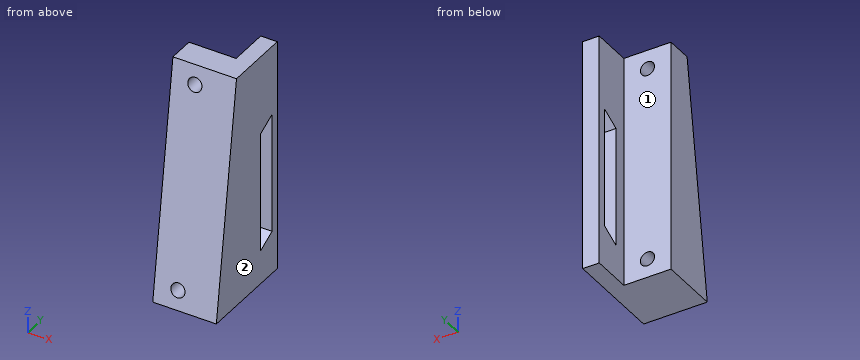
Autodesk Inventor part; units mm, degrees
ref_plane "YZ Plane" through (0, 0, 0) normal (1, 0, 0) x (0, 1, 0)
ref_plane "XZ Plane" through (0, 0, 0) normal (0, 1, 0) x (-1, 0, 0)
ref_plane "XY Plane" through (0, 0, 0) normal (0, 0, 1) x (1, 0, 0)
sketch "Sketch1" plane through (0, 0, 0) normal (0, 1, 0) x (-1, 0, 0)
  line L0 (0, 0) -> (20, 0)
  line L1 (20, 0) -> (20, -99)
  line L2 (20, -99) -> (0, -99)
  line L3 (0, -99) -> (0, 0)
  line L4 (10, 0) -> (10, -8)
  circle A0 centre (10, -8) radius 3
  line L5 (10, -99) -> (10, -91)
  circle A1 centre (10, -91) radius 3
  line L6 (0, -99) -> (-7, -99)
  line L7 (-7, -99) -> (-7, 0)
  line L8 (-7, 0) -> (0, 0)
  line L9 (0, 0) -> (0, -99)
  dimension "d0" = 20
  dimension "d1" = 99
  dimension "d2" = 8
  dimension "d3" = 6
  dimension "d4" = 8
  dimension "d5" = 6
  dimension "d8" = 7
extrude "Extrusion1" add sketch "Sketch1" along normal blind 25 contours L0 L1 L2 L3
extrude "Extrusion2" add sketch "Sketch1" along normal blind 42 contours L3 L6 L7 L8
sketch "Sketch2" plane through (0, 25, 0) normal (-1, 0, 0) x (0, 0, 1)
  line L0 (-84.6677, 5.4134) -> (-33.6677, 5.4134)
  line L1 (-33.6677, 5.4134) -> (-33.6677, 13.4134)
  line L2 (0, 17) -> (-99, 17)
  line L3 (-33.6677, 13.4134) -> (-29.6677, 13.4134)
  line L4 (-29.6677, 13.4134) -> (-80.6677, 13.4134)
  line L5 (-80.6677, 13.4134) -> (-84.6677, 5.4134)
  line L6 (-29.6677, 13.4134) -> (-33.6677, 5.4134)
  point P0 (0, -25)
  point P1 (-33.6677, 13.4134)
  dimension "d11" = 51
  dimension "d12" = 8
  dimension "d13" = 4
  dimension "d14" = 51
extrude "Extrusion3" cut sketch "Sketch2" against normal through all
sketch "Sketch3" plane through (-20, 0, -99) normal (-1, 0, 0) x (0, 0, 1)
  line L0 (0, 0) -> (99, 13.9135)
  line L1 (99, 0) -> (99, 42)
  line L2 (0, 0) -> (99.9729, 0) construction
  line L3 (99, 13.9135) -> (99, 0)
  line L4 (99, 0) -> (0, 0)
  dimension "d17" = 8
extrude "Extrusion4" cut sketch "Sketch3" against normal through all
properties part number "Podkladki_pod_laptopa"
The model under review builds one solid part; all positions refer to its coordinate system, in mm. Face numbers are marked on the shaded views. A direction names the side the tool comes from. Round coordinates to 2 decimals unless told otherwise and drop trailing zeros. Order: outer loops, then holes, each group sorted by start corner. A loop starts at its lowest first (then second) coordinate and runs counter-clockwise, first axis right, second up. Notation, with made-up numbers: (51.5, 26.25) -> (58.5, 26.25) arc R19 ccw to (58.5, 42.25) -> close; hole circle Ø4 at (61, -36). An arc over 180 degrees is marked (long way). Use a Markdown table: item, result.
Q1. Tool access review of the marked faces 1 and 2: name each direction out of +Z, -Z, +X, -X, +Y, -Y from which nothing blocks a thin tool from reaching the whole face with its end or side.
Values:
| item | result |
|---|---|
| face 1 | +Z, -Z, -X, +Y |
| face 2 | +Z, -Z, +X, +Y, -Y |
Q2. Clearance check with flat-ended pins moving along their axes: P1, Ø6, axis at x = -0.5, z = -38.5, coming from the -Y side; P2, Ø6, axis at x = 3, z = -15.5, coming from the -Y side; P3, Ø1, axis at y = 29, z = -50, coming from the -X side; P4, Ø6, axis at x = 0.5, y = 29.5, coming from the +Z side. State where each tip first meets the part, or that it passes through.
Values:
| item | result |
|---|---|
| P1 | stops at y = 8.08 |
| P2 | stops at y = 11.31 |
| P3 | stops at x = 0 |
| P4 | stops at z = 0 |
Q3. We need section A-A on x = 4.5. Write out the cut boundary in (y, z), then the cut area to 3 significant figures.
Values:
| item | result |
|---|---|
| outline | (0, -99) -> (42, -99) -> (42, 0) -> (13.91, 0) -> close; hole (30.41, -84.67) -> (38.41, -80.67) -> (38.41, -29.67) -> (30.41, -33.67) -> close |
| area | 3,060 mm^2 |
Q4. For line 1 (X direction, y = 15.25, z = -91); line 2 (Z direction, x = -12.5, y = 18); line 3 (Y direction, x = 1.25, z = -81), list the stretches that pass through material, from the lowest coordinate up.
Values:
| item | result |
|---|---|
| line 1 | x = -20 to -13, -7 to 7 |
| line 2 | z = -99 to -92.66, -89.34 to -9.66, -6.34 to 0 |
| line 3 | y = 2.53 to 30.41, 37.75 to 42 |
Q5. We need section C-C on y = 32.5. Write out the cut boundary in (x, z).
Values:
| item | result |
|---|---|
| outline | (0, -99) -> (7, -99) -> (7, -83.62) -> (0, -83.62) -> close; (0, -32.62) -> (7, -32.62) -> (7, 0) -> (0, 0) -> close |
Q6. We need section D-D on x = -10. Write out the cut boundary in (y, z).
Values:
| item | result |
|---|---|
| outline | (0, -99) -> (25, -99) -> (25, -94) -> (0.7, -94) -> close; (1.55, -88) -> (25, -88) -> (25, -11) -> (12.37, -11) -> close; (13.21, -5) -> (25, -5) -> (25, 0) -> (13.91, 0) -> close |
Q7. We need section B-B on z = -91. Write out the cut boundary in (x, y).
Values:
| item | result |
|---|---|
| outline | (-20, 1.12) -> (-13, 1.12) -> (-13, 25) -> (-20, 25) -> close; (-7, 1.12) -> (7, 1.12) -> (7, 42) -> (0, 42) -> (0, 25) -> (-7, 25) -> close |
